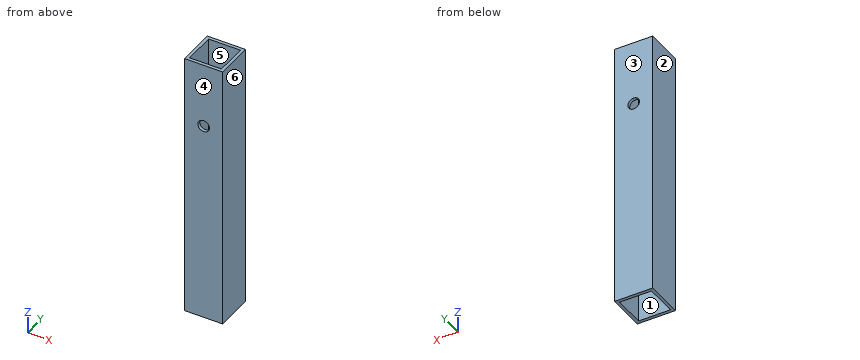
from build123d import *

# Parameters (mm, degrees)
SKETCH1_W                = 19.05
SKETCH1_H                = 19.05
SKETCH1_W_2              = 15.875
SKETCH1_H_2              = 15.875
BOSS_EXTRUDE1_DEPTH      = 66.951599904
SKETCH2_R                = 2.8956
BASEPLATEMOUNTHOLE_DEPTH = 71.25770317


with BuildPart() as part:
    # Sketch1 → Boss-Extrude1 (new, symmetric)
    with BuildSketch(Plane(origin=(0, 0, 0), x_dir=(0, -1, 0), z_dir=(0, 0, 1))):
        Rectangle(SKETCH1_W, SKETCH1_H)
        Rectangle(SKETCH1_W_2, SKETCH1_H_2, mode=Mode.SUBTRACT)
    extrude(amount=BOSS_EXTRUDE1_DEPTH, both=True)

    # Sketch2 → BasePlateMountHole (cut, through all)
    with BuildSketch(Plane(origin=(0, 9.525, 0), x_dir=(1, 0, 0), z_dir=(0, 1, 0))):
        with Locations(Location((0, -34.648400096, 0), (0, 0, 180))):
            Circle(SKETCH2_R)
    extrude(amount=-BASEPLATEMOUNTHOLE_DEPTH, mode=Mode.SUBTRACT)


solid = part.part
Can you work these out from the model? Positions are in its coordinate system, mm. Face numbers are marked on the shaded views. A direction names the side the tool comes from. Round coordinates to 2 decimals unless told otherwise and drop trailing zeros. Loops run counter-clockwise (first coordinate to the right, second up) from the corner with the lowest first, then second, coordinate; pieces in that order, holes last. Notation, with made-up numbers: (-12.75, -21.75) - (6.25, -21.75) arc R18 ccw to (6.25, -13.75) - close; hole circle Ø10 at (15, 71). An arc over 180 degrees is marked (long way). Write item = value, one per line. Start each with the question number.
(1) If we section it at D-D (z = 14.5): Please give me the cut outline in (x, y) (1 decimal).
(2) If we section it at C-C (x = 0): Please give me the cut outline in (y, z) (1 decimal), and give its area (3 significant figures).
(3) If I drill on probe 1 along X at (y, z) = (3.75, -2) (1 decimal); probe 2 along Z at (x, y) = (0, 8.65), over which ranges is the centre line in solid material (lowest first)? Write a range as [from, to].
(4) For P1, Ø6, axis at x = 6, y = -5.5, coming from the +Z side, with a flat end and sliding along its axis, tell me the tip position at first contact or that it passes through.
(5) For the marked faces 1 and 2, which set-ups out of +Z, -Z, +X, -X, +Y, -Y let a thin tool reach every point of the face, with its end or its side?
(6) If we mould it in two halves opening along Y, with no side actions, what happens to the marked faces 3, 4, 5 and 6? For each: released by +Y, released by -Y, zero draft, split by the parting line, or undercut.
(7) If we section it at A-A (x = 6.5): Please give me the cut outline in (y, z) (1 decimal), and give its area (3 significant figures).
Ans:
q1.outline = (-9.5, -9.5) - (9.5, -9.5) - (9.5, 9.5) - (-9.5, 9.5) - close; hole (-7.9, -7.9) - (7.9, -7.9) - (7.9, 7.9) - (-7.9, 7.9) - close
q2.outline = (-9.5, -67) - (-7.9, -67) - (-7.9, 31.8) - (-9.5, 31.8) - close; (-9.5, 37.5) - (-7.9, 37.5) - (-7.9, 67) - (-9.5, 67) - close; (7.9, -67) - (9.5, -67) - (9.5, 31.8) - (7.9, 31.8) - close; (7.9, 37.5) - (9.5, 37.5) - (9.5, 67) - (7.9, 67) - close
q2.area = 407 mm²
q3.probe_1 = [-9.5, -7.9], [7.9, 9.5]
q3.probe_2 = [-66.95, 31.75], [37.54, 66.95]
q4.P1 = 66.95
q5.face_1 = +Z, -Z
q5.face_2 = +Z, -Z, -X, +Y, -Y
q6.face_3 = released by +Y
q6.face_4 = released by -Y
q6.face_5 = undercut
q6.face_6 = zero draft
q7.outline = (-9.5, -67) - (-7.9, -67) - (-7.9, 67) - (-9.5, 67) - close; (7.9, -67) - (9.5, -67) - (9.5, 67) - (7.9, 67) - close
q7.area = 425 mm²
